from build123d import *

# Parameters (mm, degrees)
F0_W     = 6.35
F0_H     = 6.35
F0_W_2   = 88.9
F1_DEPTH = 3.175


with BuildPart() as f1:
    # F0 (on Top) → F1 (new body)
    with BuildSketch(Plane.XY):
        with Locations((-43.360994, 113.999984)):
            Rectangle(F0_W, F0_H)
        with Locations((4.264006, 113.999984)):
            Rectangle(F0_W_2, F0_H)
        Polygon((-40.185994, 110.824984), (-46.535994, 110.824984), (-46.535994, -3.475016), (-40.185994, -3.475016), (-40.185994, -0.300016), (48.714006, -0.300016), (48.714006, -3.475016), (55.064006, -3.475016), (55.064006, 110.824984), (48.714006, 110.824984), (48.714006, 107.649984), (-40.185994, 107.649984), align=None)
        with Locations((51.889006, 113.999984)):
            Rectangle(F0_W, F0_H)
        with Locations((-43.360994, -6.650016)):
            Rectangle(F0_W, F0_H)
        Polygon((48.714006, -3.475016), (-40.185994, -3.475016), (-40.185994, -9.825016), (4.264006, -9.825016), (48.714006, -9.825016), align=None)
        with Locations((51.889006, -6.650016)):
            Rectangle(F0_W, F0_H)
    extrude(amount=F1_DEPTH)


solid = f1.part
For this review, take the finished solid that the model builds, in its own axes (mm). A direction names the side the tool comes from. Coordinates: 2 decimals unless noted, no trailing zeros. Order: outer loops, then holes, each group sorted by start corner. A loop starts at its lowest first (then second) coordinate and runs counter-clockwise, first axis right, second up. Notation, with made-up numbers: (86.5, 9) -> (120.5, 9) arc R20 cw to (120.5, 24) -> close; hole circle Ø4 at (-37, 73). An arc over 180 degrees is marked (long way). Return JSON: item names as keys, results as strings.
1. Machinability: for faces 5 (the flat face through (48.714, -2, 2)), 6 (the flat face through (4, 55, 3.175)), which of the approach directions +Z, -Z, +X, -X, +Y, -Y give a long, thin tool a straight path to every point of the face, cutting with its end or side? Answer none if there is none.
Answer block:
{"face 5": "+Z, -Z", "face 6": "+Z, +X, -X, +Y, -Y"}
2. We need section B-B on x = -19.5. Write out the cut boundary in (y, z) (3 decimals).
Answer block:
{"outline": "(-9.825, 0) -> (-3.475, 0) -> (-3.475, 3.175) -> (-9.825, 3.175) -> close; (-0.3, 0) -> (107.65, 0) -> (107.65, 3.175) -> (-0.3, 3.175) -> close; (110.825, 0) -> (117.175, 0) -> (117.175, 3.175) -> (110.825, 3.175) -> close"}
3. The part is to be moulded in two halves that separate along Y. For faces 1 (the flat face through (5, 117.175, 2)), 2 (the flat face through (4, -0.3, 2)), 3 (the flat face through (-40.186, 109, 2)), 4 (the flat face through (-46.536, 55, 2)), say which applies: +Y half, -Y half, draft (parallel to the pull), parting line (faces both ways), or undercut.
Answer block:
{"face 1": "+Y half", "face 2": "undercut", "face 3": "undercut", "face 4": "draft"}
4. We need section A-A on z = 0.65. Write out the cut boundary in (x, y).
Answer block:
{"outline": "(-46.54, -9.83) -> (55.06, -9.83) -> (55.06, 117.17) -> (-46.54, 117.17) -> close; hole (-40.19, -3.48) -> (48.71, -3.48) -> (48.71, -0.3) -> (-40.19, -0.3) -> close; hole (-40.19, 107.65) -> (48.71, 107.65) -> (48.71, 110.82) -> (-40.19, 110.82) -> close"}
5. For line 1 (Y direction, x = 26, z = 2.9); line 2 (X direction, y = -0.5, z = 2.2), list the stretches that pass through material, from the lowest coordinate up. Write a range as from..to.
Answer block:
{"line 1": "-9.83..-3.48, -0.3..107.65, 110.82..117.17", "line 2": "-46.54..-40.19, 48.71..55.06"}
